Check sheet for the modelled part. Datum: model origin and axes. Units: mm. A direction names the side the tool comes from. Round coordinates to 2 decimals unless told otherwise and drop trailing zeros. Order: outer loops, then holes, each group sorted by start corner. A loop starts at its lowest first (then second) coordinate and runs counter-clockwise, first axis right, second up.
from build123d import *

# Parameters (mm, degrees)
F0_R     = 30
F1_DEPTH = 80
F2_R     = 25
F3_DEPTH = 40
F4_R     = 4.99999
F5_R     = 5
F6_R     = 10


# Not quite as in the source:
# - a fillet or chamfer is up to 0.001 mm smaller than in the source, because OpenCascade refuses the exact size


with BuildPart() as f1:
    # F0 (on Top) → F1 (new body)
    with BuildSketch(Plane.XY):
        Circle(F0_R)
    extrude(amount=F1_DEPTH)

    # F2 (on face) → F3 (join)
    with BuildSketch(Plane.XY.offset(80)):
        Circle(F2_R)
    extrude(amount=F3_DEPTH)

    # F4 (radius 5 in the source; OpenCascade refuses exactly that, so slightly less here)
    f4_edges = [f1.edges().sort_by_distance(p)[0] for p in [
        (-30, 0, 80),
    ]]
    fillet(f4_edges, radius=F4_R)

    # F5
    f5_edges = [f1.edges().sort_by_distance(p)[0] for p in [
        (-30, 0, 0),
    ]]
    fillet(f5_edges, radius=F5_R)

    # F6
    f6_edges = [f1.edges().sort_by_distance(p)[0] for p in [
        (-25, 0, 120),
    ]]
    fillet(f6_edges, radius=F6_R)


solid = f1.part
1) Scan lines: line 1 (Y direction, x = 0, z = 96.5); line 2 (X direction, y = -9, z = 69); line 3 (Y direction, x = 12, z = 82). Record each from-to range of solid material in increasing order.
2) Sectioned sample at D-D on z = 99.5. Record the cut outline in (x, y), and give its area (3 significant figures).
3) Set-up check for faces 1 (the face through (23.846, 7.509, 94.79)), 2 (the face through (0, 0, 120)): record each of +Z, -Z, +X, -X, +Y, -Y from which the full face is reachable in a straight line by a thin tool's end or side.
4) Gauge pin test, flat ends, axial feed: pin 1 (8 mm diameter, centred on x = -20.5, y = -8.5, fed in from +Z); pin 2 (2 mm diameter, centred on x = -23, z = 73.5, fed in from -Y); pin 3 (5 mm diameter, centred on x = 13.5, y = -13, fed in from +Z). Record the tip position at first contact, or that the pin passes through.
5) Sectioned sample at C-C on z = 32.5. Record the cut outline in (x, y).
Values found:
1. line 1: y = -25 to 25
1. line 2: x = -28.62 to 28.62
1. line 3: y = -21.93 to 21.93
2. outline: circle Ø50 at (0, 0)
2. area: 1,960 mm2
3. face 1: +Z
3. face 2: +Z, +X, -X, +Y, -Y
4. pin 1: stops at z = 119.48
4. pin 2: stops at y = -20.4
4. pin 3: stops at z = 119.92
5. outline: circle Ø60 at (0, 0)
